Check sheet for the modelled part. Datum: model origin and axes. Units: mm. Face numbers are marked on the shaded views. Give positions to 0.01 mm unless a question says otherwise; leave off trailing zeros. Write each loop counter-clockwise with the first axis right and the second up, starting at its lowest first coordinate (ties: lowest second). Pieces come first, ordered by that corner, then holes. Notation, with made-up numbers: (1.25, 87.5) -> (45.25, 87.5) arc R21 ccw to (45.25, 104.5) -> close; hole circle Ø6 at (61.25, 66). An arc over 180 degrees is marked (long way). Answer as a JSON object with one key per item and string values.
from build123d import *

# Parameters (mm, degrees)
CROQUIS1_R                   = 6
SALIENTE_EXTRUIR1_DEPTH      = 40
CROQUIS2_R                   = 1.75
CORTAR_EXTRUIR1_DEPTH        = 7.5
SALIENTE_EXTRUIR2_DEPTH      = 2
SALIENTE_EXTRUIR2_DEPTH_BACK = 3.2
CROQUIS3_R                   = 27.5
CORTAR_EXTRUIR2_DEPTH        = 58.240719845
CORTAR_EXTRUIR2_DEPTH_BACK   = 5.2
CROQUIS5_R                   = 2.15
REDONDEO1_R                  = 1


with BuildPart() as part:
    # Croquis1 → Saliente-Extruir1 (new body)
    with BuildSketch(Plane.XY):
        Circle(CROQUIS1_R)
        with BuildLine():
            Line((-1.8, 2.585053191), (1.8, 2.585053191))
            ThreePointArc((1.8, 2.585053191), (0, -3.15), (-1.8, 2.585053191))
        make_face(mode=Mode.SUBTRACT)
    extrude(amount=SALIENTE_EXTRUIR1_DEPTH)

    # Croquis2 → Cortar-Extruir1 (cut)
    with BuildSketch(Plane(origin=(0, 2.585053191, 0), x_dir=(1, 0, 0), z_dir=(0, 1, 0))):
        with Locations((0, -36.75)):
            Circle(CROQUIS2_R)
        with Locations((0, -31.25)):
            Circle(CROQUIS2_R)
    extrude(amount=CORTAR_EXTRUIR1_DEPTH, mode=Mode.SUBTRACT)

    # Croquis3 → Saliente-Extruir2 (add, two sides: drawn at the far end of the back side and taken through both)
    with BuildSketch(Plane(origin=(0, 0, 0), x_dir=(-1, 0, 0), z_dir=(0, 0, -1)).offset(-SALIENTE_EXTRUIR2_DEPTH_BACK)):
        Circle(CROQUIS3_R)
    extrude(amount=SALIENTE_EXTRUIR2_DEPTH + SALIENTE_EXTRUIR2_DEPTH_BACK)

    # Croquis5 → Cortar-Extruir2 (cut, two sides: drawn at the far end of the back side and taken through both)
    with BuildSketch(Plane(origin=(0, 0, -2), x_dir=(-1, 0, 0), z_dir=(0, 0, -1)).offset(-CORTAR_EXTRUIR2_DEPTH_BACK)):
        with Locations(Location((-20, 0, 0), (0, 0, 180))):
            Circle(CROQUIS5_R)
        with Locations(Location((20, 0, 0), (0, 0, 180))):
            Circle(CROQUIS5_R)
    extrude(amount=CORTAR_EXTRUIR2_DEPTH + CORTAR_EXTRUIR2_DEPTH_BACK, mode=Mode.SUBTRACT)

    # Redondeo1
    redondeo1_edges = [part.edges().sort_by_distance(p)[0] for p in [
        (27.5, 0, 3.2),
        (27.5, 0, -2),
    ]]
    fillet(redondeo1_edges, radius=REDONDEO1_R)


solid = part.part
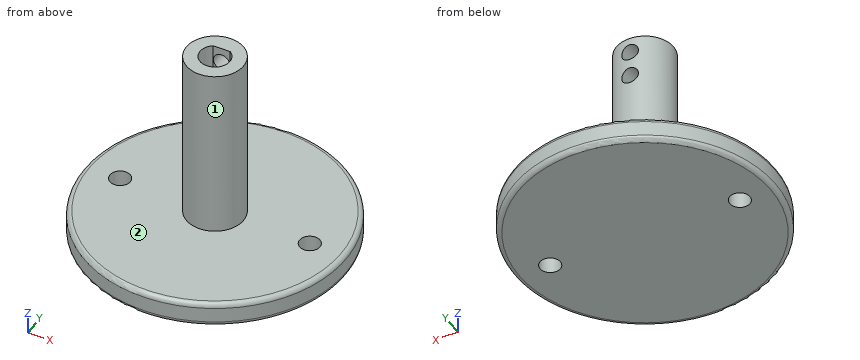
1. Go/stop test with flat-tipped pins: P1, Ø1, axis at y = 8, z = 7, coming from the +X side; P2, Ø7, axis at x = -20, y = 0, coming from the +Z side; P3, Ø5, axis at x = 20, y = 0, coming from the -Z side; P4, Ø3, axis at x = 0, z = 31.25, coming from the -Y side. Record where each tip stops, or that it passes through.
Determined:
{"P1": "through", "P2": "z = 3.2", "P3": "z = -2", "P4": "y = -6"}
2. Scan lines: L1, parallel to Z at x = 0, y = 3.4; L2, parallel to Y at x = 0, z = 23.5; L3, parallel to Z at x = 16, y = -9.5. Record each from-to range of solid material in increasing order. Write a range as [from, to].
Determined:
{"L1": "[-2, 29.5], [33, 35], [38.5, 40]", "L2": "[-6, -3.15], [2.59, 6]", "L3": "[-2, 3.2]"}
3. Sectioned sample at A-A, the plane x = 0. Enter the section's corners in (y, z).
Determined:
{"outline": "(-27.5, -1) arc R1 ccw to (-26.5, -2) -> (26.5, -2) arc R1 ccw to (27.5, -1) -> (27.5, 2.2) arc R1 ccw to (26.5, 3.2) -> (6, 3.2) -> (6, 29.5) -> (2.59, 29.5) -> (2.59, 3.2) -> (-3.15, 3.2) -> (-3.15, 40) -> (-6, 40) -> (-6, 3.2) -> (-26.5, 3.2) arc R1 ccw to (-27.5, 2.2) -> close; (2.59, 33) -> (6, 33) -> (6, 35) -> (2.59, 35) -> close; (2.59, 38.5) -> (6, 38.5) -> (6, 40) -> (2.59, 40) -> close"}
4. Mould release check, pull along Y, two halves, no side actions. Record for the marked faces 1 and 2: released by +Y, released by -Y, zero draft, split by the parting line, or undercut.
Determined:
{"face 1": "split by the parting line", "face 2": "zero draft"}
5. Sectioned sample at C-C, the plane y = 4.5. State how many separate pieces and enclosed holes the cut face has, plus the area to 3 significant figures.
Determined:
{"separate pieces": "1", "enclosed holes": "2", "area": "554 mm^2"}
6. Sectioned sample at D-D, the plane z = 31.25. Enter the section's corners in (x, y), plus the area to 3 significant figures.
Determined:
{"outline": "(-1.8, 2.59) -> (-1.75, 2.59) -> (-1.75, 5.74) arc R6 ccw (long way) to (1.75, 5.74) -> (1.75, 2.59) -> (1.8, 2.59) arc R3.15 cw (long way) to start", "area": "71.7 mm^2"}
7. Sectioned sample at B-B, the plane z = 12.5. Enter the section's corners in (x, y), plus the area to 3 significant figures.
Determined:
{"outline": "circle Ø12 at (0, 0); hole (-1.8, 2.59) arc R3.15 ccw (long way) to (1.8, 2.59) -> close", "area": "83.3 mm^2"}
